Geometry: final body of the model. Coordinates: model frame, mm. Face numbers are marked on the shaded views. A direction names the side the tool comes from. Round coordinates to 2 decimals unless told otherwise and drop trailing zeros. Write each loop counter-clockwise with the first axis right and the second up, starting at its lowest first coordinate (ties: lowest second). Pieces come first, ordered by that corner, then holes.
from build123d import *

# Parameters (mm, degrees)
SALIENTE_EXTRUIR1_DEPTH = 30
CROQUIS3_W              = 4.89350096
CROQUIS3_H              = 4.01782184
SALIENTE_EXTRUIR2_DEPTH = 3
SALIENTE_EXTRUIR3_DEPTH = 41.5
REDONDEO2_R             = 3


with BuildPart() as part:
    # Croquis1 → Saliente-Extruir1 (new body)
    with BuildSketch(Plane(origin=(0, 0, 0), x_dir=(1, 0, 0), z_dir=(0, 1, 0))):
        with BuildLine():
            Line((-6, 8), (6, 8))
            ThreePointArc((6, 8), (10.242640687, 6.242640687), (12, 2))
            Line((12, 2), (12, -2))
            ThreePointArc((12, -2), (10.242640687, -6.242640687), (6, -8))
            Line((6, -8), (-6, -8))
            ThreePointArc((-6, -8), (-10.242640687, -6.242640687), (-12, -2))
            Line((-12, -2), (-12, 2))
            ThreePointArc((-12, 2), (-10.242640687, 6.242640687), (-6, 8))
        make_face()
        with BuildLine():
            Line((-6, -5), (6, -5))
            ThreePointArc((6, -5), (8.121320344, -4.121320344), (9, -2))
            Line((9, -2), (9, 2))
            ThreePointArc((9, 2), (8.121320344, 4.121320344), (6, 5))
            Line((6, 5), (-6, 5))
            ThreePointArc((-6, 5), (-8.121320344, 4.121320344), (-9, 2))
            Line((-9, 2), (-9, -2))
            ThreePointArc((-9, -2), (-8.121320344, -4.121320344), (-6, -5))
        make_face(mode=Mode.SUBTRACT)
    extrude(amount=SALIENTE_EXTRUIR1_DEPTH)

    # Croquis3 → Saliente-Extruir2 (add)
    with BuildSketch(Plane(origin=(0, 0, -8), x_dir=(-1, 0, 0), z_dir=(0, 0, -1))):
        with Locations((0, 15)):
            Rectangle(CROQUIS3_W, CROQUIS3_H)
    extrude(amount=SALIENTE_EXTRUIR2_DEPTH)

    # Croquis7 → Saliente-Extruir3 (add, symmetric)
    with BuildSketch(Plane(origin=(0, 17.00891092, 0), x_dir=(1, 0, 0), z_dir=(0, 1, 0))):
        Polygon((-2.44675048, 11), (2.44675048, 11), (25.428083774, 30.283628291), (33.597669299, 42.86368681), (31.920328163, 43.95296488), (23.913536336, 31.623586673), (1.718810011, 13), (-1.718810011, 13), (-23.913536336, 31.623586673), (-31.920328163, 43.95296488), (-33.597669299, 42.86368681), (-25.428083774, 30.283628291), align=None)
    extrude(amount=SALIENTE_EXTRUIR3_DEPTH, both=True)

    # Redondeo2
    # the kernel refuses this fillet: 3 mm, written as the material it adds along each edge
    with BuildSketch(Plane(origin=(-23.913536336, -24.49108908, -31.623586673), x_dir=(0.7660444431189832, 0, 0.6427876096865331), z_dir=(0, 1, 0)), Plane(origin=(23.913536336, -24.49108908, -31.623586673), x_dir=(0.5446390350150309, 0, -0.8386705679454215), z_dir=(0, 1, 0))) as redondeo2_piece_1:
        with BuildLine():
            CenterArc((REDONDEO2_R * 0.149451001349, REDONDEO2_R), REDONDEO2_R, 253, 17)
            Line((-REDONDEO2_R * 0.142920703374, REDONDEO2_R * 0.043695244037), (0, 0))
            Line((0, 0), (REDONDEO2_R * 0.149451001349, 0))
        make_face()
    extrude(amount=83)
    with BuildSketch(Plane(origin=(1.718810011, -24.49108908, -13), x_dir=(0.7660444431189833, 0, -0.6427876096865328), z_dir=(0, 1, 0)), Plane(origin=(-1.718810011, -24.49108908, -13), x_dir=(1, 0, 0), z_dir=(0, 1, 0))) as redondeo2_piece_2:
        with BuildLine():
            CenterArc((REDONDEO2_R * 0.363970234266, REDONDEO2_R), REDONDEO2_R, 230, 40)
            Line((-REDONDEO2_R * 0.27881737542, REDONDEO2_R * 0.233955556881), (0, 0))
            Line((0, 0), (REDONDEO2_R * 0.363970234266, 0))
        make_face()
    extrude(amount=83)
    # the kernel refuses this fillet: 3 mm, written as the material it takes off along each edge
    with BuildSketch(Plane(origin=(31.920328163, -31.562156891, -43.95296488), x_dir=(0.8386705679454225, 0, 0.5446390350150296), z_dir=(0, 1, 0))) as redondeo2_2_piece_1:
        with BuildLine():
            CenterArc((3, -2.828427125), REDONDEO2_R, 109.471220634, 70.528779366)
            Line((0, -2.828427125), (0, 0))
            Line((0, 0), (2, 0))
        make_face()
    extrude(amount=97.142135624, mode=Mode.SUBTRACT)
    with BuildSketch(Plane(origin=(-31.920328163, -31.562156891, -43.95296488), x_dir=(0.5446390350150306, 0, 0.8386705679454217), z_dir=(0, 1, 0))) as redondeo2_2_piece_2:
        with BuildLine():
            CenterArc((2.828427125, -3), REDONDEO2_R, 90, 70.528779366)
            Line((0, -2), (0, 0))
            Line((0, 0), (2.828427125, 0))
        make_face()
    extrude(amount=97.142135624, mode=Mode.SUBTRACT)


solid = part.part
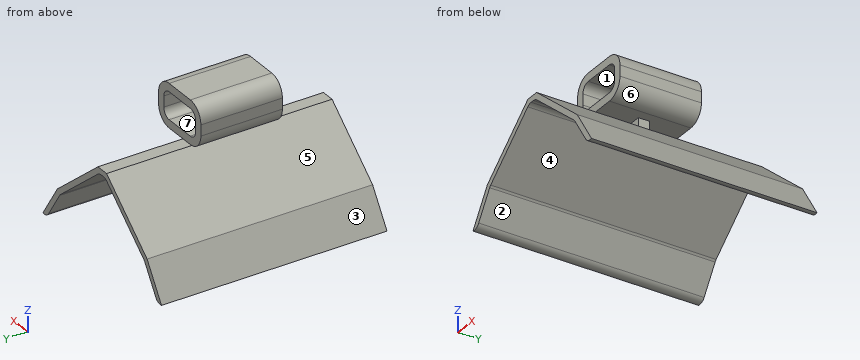
1) First-contact query: P1, Ø5.5, axis at x = 0, y = -4.5, coming from the +Z side; P2, Ø2, axis at y = 14.5, z = 1, coming from the -X side; P3, Ø1.5, axis at x = 6, y = 19, coming from the -Z side; P4, Ø8, axis at x = -15, z = -27, coming from the -Y side. Flat tips, straight axial feed; report the tip coordinate or a pass-through.
2) Draft query along Z for the marked faces 1, 2 and 3. Return one class per face: pulls with the +Z half, pulls with the -Z half, needs draft (parallel to the pull), parting line crosses it, or undercut.
3) Section B-B on x = -10. Output: boundary loops of the cut face in (y, z).
4) Reachability of the marked faces 4, 5, 6 and 7 from +Z, -Z, +X, -X, +Y, -Y: full face, straight path, thin tool, end or side. Return the list, or none.
5) Section D-D on y = -15.5. Output: boundary loops of the cut face in (x, z).
6) Section C-C on z = -24.5. Output: boundary loops of the cut face in (x, y), plus the area to 4 significant figures.
7) Section A-A on y = 20. State how many separate pieces and enclosed holes the cut face has, plus the area to 3 significant figures.
8) Line query: probe 1 along Z at (x, y) = (0.5, 19.5); probe 2 along X at (y, z) = (34, -27.5); probe 3 along X at (y, z) = (0.5, -39). Output: solid intervals per line, ascending.
Filled in:
1. P1: stops at z = -11
1. P2: stops at x = -12
1. P3: stops at z = -17.22
1. P4: stops at y = -24.49
2. face 1: undercut
2. face 2: pulls with the -Z half
2. face 3: pulls with the +Z half
3. outline: (-24.49, -19.95) - (58.51, -19.95) - (58.51, -17.34) - (-24.49, -17.34) - close; (0, -6.47) - (30, -6.47) - (30, 6.47) - (0, 6.47) - close
4. face 4: -Z, +Y, -Y
4. face 5: -X, +Y, -Y
4. face 6: +X, +Y, -Y
4. face 7: +Y, -Y
5. outline: (-33.6, -42.86) arc R3 ccw to (-30.38, -41.58) - (-24.16, -32) arc R3 cw to (-23.57, -31.34) - (-2.56, -13.7) arc R3 cw to (-0.63, -13) - (0.63, -13) arc R3 cw to (2.56, -13.7) - (23.57, -31.34) arc R3 cw to (24.16, -32) - (30.38, -41.58) arc R3 ccw to (33.6, -42.86) - (25.43, -30.28) - (2.45, -11) - (-2.45, -11) - (-25.43, -30.28) - close
6. outline: (-18.54, -24.49) - (-15.42, -24.49) - (-15.42, 58.51) - (-18.54, 58.51) - close; (15.42, -24.49) - (18.54, -24.49) - (18.54, 58.51) - (15.42, 58.51) - close
6. area: 516.5 mm2
7. separate pieces: 2
7. enclosed holes: 1
7. area: 364 mm2
8. probe 1: z = -13 to -11, -8 to -5, 5 to 8
8. probe 2: x = -22.11 to -19, 19 to 22.11
8. probe 3: x = -31.09 to -28.7, 28.7 to 31.09
